Work out the finished part from the listing and answer in its coordinate system (mm). Face numbers are marked on the shaded views. Coordinates: 2 decimals unless noted, no trailing zeros. Loops run counter-clockwise (first coordinate to the right, second up) from the corner with the lowest first, then second, coordinate; pieces in that order, holes last. Notation, with made-up numbers: (63.25, -28) -> (102.25, -28) arc R14 cw to (102.25, -16) -> close; hole circle Ø11 at (44, 59). An arc over 180 degrees is marked (long way). Use a Markdown table: item, result.
from build123d import *

# Parameters (mm, degrees)
BOSS_EXTRUDE1_DEPTH         = 120
BOSS_EXTRUDE1_DEPTH_BACK    = 120
FILLET1_R                   = 2
HOLE1_D                     = 4
HOLE1_CBORE_D               = 8
HOLE1_CBORE_DEPTH           = 3.1
HOLE1_ON_FACE_2_D           = 4
HOLE1_ON_FACE_2_CBORE_D     = 8
HOLE1_ON_FACE_2_CBORE_DEPTH = 3.1
HOLE1_ON_FACE_3_D           = 4
HOLE1_ON_FACE_3_CBORE_D     = 8
HOLE1_ON_FACE_3_CBORE_DEPTH = 3.1
HOLE1_ON_FACE_4_D           = 4
HOLE1_ON_FACE_4_CBORE_D     = 8
HOLE1_ON_FACE_4_CBORE_DEPTH = 3.1
HOLE1_ON_FACE_5_D           = 4
HOLE1_ON_FACE_5_CBORE_D     = 8
HOLE1_ON_FACE_5_CBORE_DEPTH = 3.1
HOLE1_ON_FACE_6_D           = 4
HOLE1_ON_FACE_6_CBORE_D     = 8
HOLE1_ON_FACE_6_CBORE_DEPTH = 3.1


with BuildPart() as part:
    # Sketch1 → Boss-Extrude1 (new, two sides: drawn at the far end of the back side and taken through both)
    with BuildSketch(Plane.XY.offset(-BOSS_EXTRUDE1_DEPTH_BACK)):
        with BuildLine():
            Line((-66.491800306, -127.729559978), (-66.491800306, -133.341068288))
            ThreePointArc((-66.491800306, -133.341068288), (0, -149), (66.491800306, -133.341068288))
            Line((66.491800306, -133.341068288), (66.491800306, -127.729559978))
            ThreePointArc((66.491800306, -127.729559978), (0, -144), (-66.491800306, -127.729559978))
        make_face()
    extrude(amount=BOSS_EXTRUDE1_DEPTH + BOSS_EXTRUDE1_DEPTH_BACK)

    # Fillet1
    fillet1_edges = [part.edges().sort_by_distance(p)[0] for p in [
        (-66.491800306, -130.535314133, 120),
        (66.491800306, -130.535314133, -120),
        (66.491800306, -130.535314133, 120),
        (-66.491800306, -130.535314133, -120),
        (66.491800306, -133.341068288, 0),
        (-66.491800306, -133.341068288, 0),
    ]]
    fillet(fillet1_edges, radius=FILLET1_R)

    # Hole1 (through all)
    with Locations(Plane(origin=(-57.019831422, -137.658050344, 111), x_dir=(-0.923879532511, 0.382683432365, 0), z_dir=(-0.382683432365, -0.923879532511, 0))):
        with Locations((0, 0)):
            CounterBoreHole(HOLE1_D / 2, HOLE1_CBORE_D / 2, HOLE1_CBORE_DEPTH)

    # Hole1 on face 2 (through all)
    with Locations(Plane(origin=(-19.448402641, -147.725284345, 111), x_dir=(-0.991444888611, 0.130525985335, 0), z_dir=(-0.130525985335, -0.991444888611, 0))):
        with Locations((0, 0)):
            CounterBoreHole(HOLE1_ON_FACE_2_D / 2, HOLE1_ON_FACE_2_CBORE_D / 2, HOLE1_ON_FACE_2_CBORE_DEPTH)

    # Hole1 on face 3 (through all)
    with Locations(Plane(origin=(19.448402641, -147.725284345, 111), x_dir=(-0.991444888611, -0.130525985335, 0), z_dir=(0.130525985335, -0.991444888611, 0))):
        with Locations((0, 0)):
            CounterBoreHole(HOLE1_ON_FACE_3_D / 2, HOLE1_ON_FACE_3_CBORE_D / 2, HOLE1_ON_FACE_3_CBORE_DEPTH)

    # Hole1 on face 4 (through all)
    with Locations(Plane(origin=(-57.019831422, -137.658050344, -111), x_dir=(-0.923879753837, 0.382682898036, 0), z_dir=(-0.382682898036, -0.923879753837, 0))):
        with Locations((0, 0)):
            CounterBoreHole(HOLE1_ON_FACE_4_D / 2, HOLE1_ON_FACE_4_CBORE_D / 2, HOLE1_ON_FACE_4_CBORE_DEPTH)

    # Hole1 on face 5 (through all)
    with Locations(Plane(origin=(0, -149, -111), x_dir=(0, 0, -1), z_dir=(0, -1, 0))):
        with Locations((0, 0)):
            CounterBoreHole(HOLE1_ON_FACE_5_D / 2, HOLE1_ON_FACE_5_CBORE_D / 2, HOLE1_ON_FACE_5_CBORE_DEPTH)

    # Hole1 on face 6 (through all)
    with Locations(Plane(origin=(57.019831422, -137.658050344, -111), x_dir=(-0.923879753837, -0.382682898036, 0), z_dir=(0.382682898036, -0.923879753837, 0))):
        with Locations((0, 0), (0, -222)):
            CounterBoreHole(HOLE1_ON_FACE_6_D / 2, HOLE1_ON_FACE_6_CBORE_D / 2, HOLE1_ON_FACE_6_CBORE_DEPTH)


solid = part.part
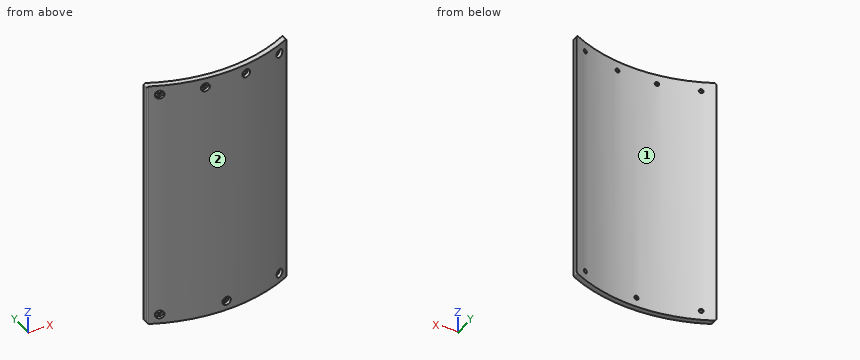
Q1. Given pin 1 Ø5 at (x, z) = (0, -111) entering from +Y; pin 2 Ø10 at (x, y) = (-5.5, -134) entering from -Z; pin 3 Ø6 at (x, z) = (32.5, 68.5) entering from -Y; pin 4 Ø8 at (x, z) = (-6, 14.5) entering from +Y, each flat-ended and moving along its own axis, determine where each tip first touches the part or whether it passes through.
Solved:
| item | result |
|---|---|
| pin 1 | y = -143.98 |
| pin 2 | through |
| pin 3 | y = -146.05 |
| pin 4 | y = -143.65 |
Q2. Determine the mould class of the marked faces 1 and 2 for opening direction X: pulls with the +X half, pulls with the -X half, needs draft (parallel to the pull), parting line crosses it, or undercut.
Solved:
| item | result |
|---|---|
| face 1 | undercut |
| face 2 | parting line crosses it |
Q3. Section C-C on x = -11.5 is taken. Determine the outline of the cut face in (y, z), and give its area (3 significant figures).
Solved:
| item | result |
|---|---|
| outline | (-148.56, -120) -> (-143.54, -120) -> (-143.54, 120) -> (-148.56, 120) -> close |
| area | 1,200 mm² |
Q4. Consider line 1 (Z direction, x = 0, y = -145.4); line 2 (Z direction, x = 0, y = -148.15); line 3 (X direction, y = -131.5, z = 60.5). Determine where each line is inside the solid, lowest interval first. Write a range as [from, to].
Solved:
| item | result |
|---|---|
| line 1 | [-120, -113], [-109, 120] |
| line 2 | [-120, -115], [-107, 120] |
| line 3 | [-66.49, -58.68], [58.68, 66.49] |
Q5. Section B-B on x = 33 is taken. Determine the outline of the cut face in (y, z), and give its area (3 significant figures).
Solved:
| item | result |
|---|---|
| outline | (-145.3, -120) -> (-140.17, -120) -> (-140.17, 120) -> (-145.3, 120) -> close |
| area | 1,230 mm² |
Q6. Section A-A on z = -72.5 is taken. Determine the outline of the cut face in (x, y), and give its area (3 significant figures).
Solved:
| item | result |
|---|---|
| outline | (-66.49, -132.1) arc R2 ccw to (-65.37, -133.89) arc R149 ccw to (65.37, -133.89) arc R2 ccw to (66.49, -132.1) -> (66.49, -127.73) arc R144 cw to (-66.49, -127.73) -> close |
| area | 690 mm² |
